Verification items for the finished model (mm, model axes). Face numbers are marked on the shaded views. A direction names the side the tool comes from. Round coordinates to 2 decimals unless told otherwise and drop trailing zeros.
from build123d import *

# Parameters (mm, degrees)
SKETCH004_R     = 20.812872
POCKET_DEPTH    = 46.345478
SKETCH005_R     = 15.581959
POCKET001_DEPTH = 5


with BuildPart() as part:
    # Sketch001 → Revolution (revolve)
    with BuildSketch(Plane.XZ):
        with BuildLine():
            Line((0, -6), (-40, -6))
            Line((-40, -6), (-55, -6))
            ThreePointArc((-40, 0), (-48.077747, -1.555632), (-55, -6))
            Line((-40, 0), (0, 0))
            Line((0, -6), (0, 0))
        make_face()
    revolve(axis=Axis((0, 0, 0), (0, 0, 1)))

    # Sketch002 (on Face4 of Revolution) → AdditiveLoft section 0
    with BuildSketch(Plane(origin=(0, 0, 0), x_dir=(-1, 0, 0), z_dir=(0, 0, 1))):
        Polygon((-6, 39.54744), (6, 39.54744), (6, 6), (39.54744, 6), (39.54744, -6), (6, -6), (6, -39.54744), (-6, -39.54744), (-6, -6), (-39.54744, -6), (-39.54744, 6), (-6, 6), align=None)
    # Sketch003 (on Face4 of Revolution) → AdditiveLoft section 1
    with BuildSketch(Plane(origin=(0, 0, 70), x_dir=(-1, 0, 0), z_dir=(0, 0, 1))):
        Polygon((-3, 14.696938), (3, 14.696938), (3, 3), (14.696938, 3), (14.696938, -3), (3, -3), (3, -14.696938), (-3, -14.696938), (-3, -3), (-14.696938, -3), (-14.696938, 3), (-3, 3), align=None)
    loft()

    # Sphere → Sphere (revolve)
    with BuildSketch(Plane(origin=(0, 0, 70), x_dir=(-1, 0, 0), z_dir=(0, 1, 0))):
        with BuildLine():
            ThreePointArc((0, -25), (25, 0), (0, 25))
            Line((0, 25), (0, -25))
        make_face()
    revolve(axis=Axis((0, 0, 70), (0, 0, 1)))

    # Sketch004 (on DatumPlane) → Pocket (cut, through all)
    with BuildSketch(Plane(origin=(0, -30.562796, 25.308346), x_dir=(-1, 0, 0), z_dir=(0, -0.942378, 0.334551))):
        with Locations((0, -52.341228)):
            Circle(SKETCH004_R)
    extrude(amount=POCKET_DEPTH, mode=Mode.SUBTRACT)

    # Sketch005 (on Face25 of Pocket) → Pocket001 (cut)
    with BuildSketch(Plane(origin=(0, -13.051994, 74.633552), x_dir=(1, 0, 0), z_dir=(0, -0.942378, 0.334551))):
        Circle(SKETCH005_R)
    extrude(amount=-POCKET001_DEPTH, mode=Mode.SUBTRACT)


solid = part.part
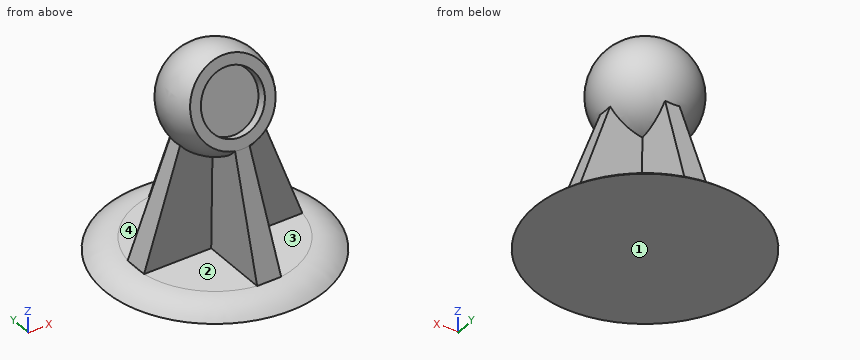
1. Release check for a two-part mould opening along Z. For the marked faces 1 and 2 record: released by +Z, released by -Z, zero draft, split by the parting line, or undercut.
2. Gauge pin test, flat ends, axial feed: P1, Ø0.5, axis at x = 40, y = -1, coming from the +Z side; P2, Ø3, axis at x = -5, z = 83, coming from the +Y side; P3, Ø1.5, axis at y = -31, z = 10, coming from the -X side. Record the tip position at first contact, or that the pin passes through.
3. Tool access check on the marked faces 3 and 4. Record the directions out of +Z, -Z, +X, -X, +Y, -Y that give a thin tool (end or side, any length) a straight path to the whole face; none if there is none.
4. Scan lines: L1, parallel to Z at x = 18.5, y = -24; L2, parallel to Z at x = -2, y = -50; L3, parallel to Z at x = -10.5, y = 13. Record each from-to range of solid material in increasing order.
Taken from the geometry:
1. face 1: released by -Z
1. face 2: undercut
2. P1: stops at z = 0
2. P2: stops at y = 21.69
2. P3: stops at x = -5.6
3. face 3: +X, -Y
3. face 4: -X, +Y
4. L1: z = -6 to 0
4. L2: z = -6 to -2.46
4. L3: z = -6 to 0, 51.41 to 88.59
